Source: CAD feature listing. Evaluate the final solid. Frame: model axes, mm. Face numbers are marked on the shaded views. A direction names the side the tool comes from. Give positions to 0.01 mm unless a question says otherwise; leave off trailing zeros. Loops run counter-clockwise (first coordinate to the right, second up) from the corner with the lowest first, then second, coordinate; pieces in that order, holes last. Notation, with made-up numbers: (-8, 26.5) -> (2, 26.5) arc R16 ccw to (2, 49.5) -> close; hole circle Ø3 at (27.5, 78.25). An arc over 180 degrees is marked (long way). Return JSON: item names as keys, results as strings. Group by question number.
```python
from build123d import *

# Parameters (mm, degrees)
F0_R     = 6
F1_DEPTH = 8
F2_DEPTH = 10
F3_R     = 6
F4_DEPTH = 20
F7_DEPTH = 8
F8_DEPTH = 8


with BuildPart() as f1:
    # F0 (on Right) → F1 (new body)
    with BuildSketch(Plane.YZ):
        with BuildLine():
            Line((-9.4280904158, 18.3333333333), (-14.1421356237, 5))
            ThreePointArc((-14.1421356237, 5), (0, -15), (14.1421356237, 5))
            Line((14.1421356237, 5), (9.4280904158, 18.3333333333))
            ThreePointArc((9.4280904158, 18.3333333333), (0, 25), (-9.4280904158, 18.3333333333))
        make_face()
        Circle(F0_R, mode=Mode.SUBTRACT)
        Circle(F0_R)
    extrude(amount=F1_DEPTH)

    # F0 (on Right) → F2 (join)
    with BuildSketch(Plane.YZ):
        Circle(F0_R)
    extrude(amount=-F2_DEPTH)

    # F3 (on face) → F4 (join)
    with BuildSketch(Plane.YZ.offset(8)):
        with Locations((0, 15)):
            Circle(F3_R)
    extrude(amount=F4_DEPTH)

    # F6: F1 across plane


with BuildPart() as f1_1:
    add(f1.part)
    add(f1.part.mirror(Plane.YZ.offset(-10)))

    # F7 (add): a face of the model
    f7_faces = [f1_1.faces().sort_by_distance(p)[0] for p in [
        (28, 0, 15),
    ]]
    extrude(f7_faces, amount=F7_DEPTH)

    # F8 (add): a face of the model
    f8_faces = [f1_1.faces().sort_by_distance(p)[0] for p in [
        (-48, 0, 15),
    ]]
    extrude(f8_faces, amount=F8_DEPTH)


solid = f1_1.part
```
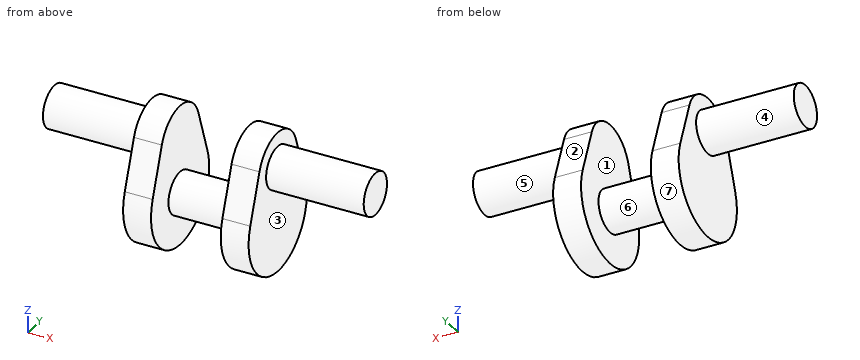
1) Material intervals for line 1 (X direction, y = -0.25, z = -8); line 2 (X direction, y = -0.25, z = 13); line 3 (Y direction, x = 21, z = 20.5), sorted ascending.
2) Contact query for flat-ended pins moving along their axis: P1, Ø8, axis at x = -6.5, z = 1, coming from the +Y side; P2, Ø1.5, axis at y = -4, z = 4, coming from the +X side; P3, Ø3, axis at y = -8, z = 5, coming from the -X side. Output: stop coordinate, or through.
3) Cut plane D-D on z = 0. Return loops of the section in (x, y).
4) Cut plane C-C on y = 0. Return loops of the section in (x, z).
5) Mould query, pull axis X, two halves, no side actions, for the marked faces 1, 2 and 3. Classes: released by +X, released by -X, zero draft, split by the parting line, or undercut.
6) Reachability of the marked faces 4, 5, 6 and 7 from +Z, -Z, +X, -X, +Y, -Y: full face, straight path, thin tool, end or side. Return the list, or none.
7) Cut plane B-B on z = 15. Return loops of the section in (x, y).
8) Cut plane A-A on y = -11. Return loops of the section in (x, z).
Calculated:
{
 "1": {"line 1": "-28 to -20, 0 to 8", "line 2": "-56 to -20, 0 to 36", "line 3": "-2.4 to 2.4"},
 "2": {"P1": "y = 6", "P2": "x = 8", "P3": "x = -28"},
 "3": {"outline": "(-28, -15) -> (-20, -15) -> (-20, -6) -> (0, -6) -> (0, -15) -> (8, -15) -> (8, 15) -> (0, 15) -> (0, 6) -> (-20, 6) -> (-20, 15) -> (-28, 15) -> close"},
 "4": {"outline": "(-56, 9) -> (-28, 9) -> (-28, -15) -> (-20, -15) -> (-20, -6) -> (0, -6) -> (0, -15) -> (8, -15) -> (8, 9) -> (36, 9) -> (36, 21) -> (8, 21) -> (8, 25) -> (0, 25) -> (0, 6) -> (-20, 6) -> (-20, 25) -> (-28, 25) -> (-28, 21) -> (-56, 21) -> close"},
 "5": {"face 1": "undercut", "face 2": "zero draft", "face 3": "released by +X"},
 "6": {"face 4": "-X", "face 5": "+X", "face 6": "none", "face 7": "+X, -X"},
 "7": {"outline": "(-56, -6) -> (-28, -6) -> (-28, -10.61) -> (-20, -10.61) -> (-20, 10.61) -> (-28, 10.61) -> (-28, 6) -> (-56, 6) -> close; (0, -10.61) -> (8, -10.61) -> (8, -6) -> (36, -6) -> (36, 6) -> (8, 6) -> (8, 10.61) -> (0, 10.61) -> close"},
 "8": {"outline": "(-28, -10.2) -> (-20, -10.2) -> (-20, 13.89) -> (-28, 13.89) -> close; (0, -10.2) -> (8, -10.2) -> (8, 13.89) -> (0, 13.89) -> close"}
}
